Design review of the part built by this model. Coordinates are the model's own, in mm. Round coordinates to 2 decimals unless told otherwise and drop trailing zeros. Loops run counter-clockwise (first coordinate to the right, second up) from the corner with the lowest first, then second, coordinate; pieces in that order, holes last. Notation, with made-up numbers: (46.25, 60) - (96.25, 60) arc R23 cw to (96.25, 95) - close; hole circle Ø7 at (18, 7.5). An arc over 180 degrees is marked (long way). Return JSON: item names as keys, results as strings. Group by question number.
from build123d import *

# Parameters (mm, degrees)
F0_W     = 50
F0_H     = 80
F1_DEPTH = 30
F2_R     = 14.968124
F3_SIZE  = 10
F4_R     = 6
F4_R_2   = 7.5
F5_DEPTH = 80.8


with BuildPart() as f1:
    # F0 (on Top) → F1 (new body)
    with BuildSketch(Plane.XY):
        with Locations((25, -40)):
            Rectangle(F0_W, F0_H)
    extrude(amount=F1_DEPTH)

    # F2
    f2_edges = [f1.edges().sort_by_distance(p)[0] for p in [
        (50, -40, 30),
    ]]
    fillet(f2_edges, radius=F2_R)

    # F3
    f3_edges = [f1.edges().sort_by_distance(p)[0] for p in [
        (0, -40, 30),
    ]]
    chamfer(f3_edges, length=F3_SIZE)

    # F4 (on face) → F5 (cut)
    with BuildSketch(Plane.XZ.offset(80)):
        with Locations((17.158328, 19.422975)):
            Circle(F4_R)
        with Locations((32.230863, 9.653739)):
            Circle(F4_R_2)
    extrude(amount=-F5_DEPTH, mode=Mode.SUBTRACT)


solid = f1.part
Q1. Add section A-A, the plane z = 12.5. State the section outline as (x, y) points, plus the area to 3 significant figures.
Q2. Add section D-D, the plane y = -22.5. State the section outline as (x, z) points.
Q3. Draft analysis for pull direction X (two halves, no side actions). For faces 1 (the cylindrical face through (19.93, -40.56, 14.1)), 2 (the flat face through (0, -41, 10)), 3 (the flat face through (50, -41, 7)), 4 (the cylindrical face through (39.385, -40.56, 11.907)), state which applies: pulls with the +X half, pulls with the -X half, needs draft (parallel to the pull), parting line crosses it, or undercut.
Q4. Insertion check: pin 1 Ø6 at (y, z) = (-43, 23.5) entering from +X. The pin has a flat end and moves straight along its axis. Give the tip position at first contact, or say it passes through.
Q5. Add section C-C, the plane x = 27. State the section outline as (y, z) points, plus the area to 3 significant figures.
Q6. For line 1 (Z direction, x = 17, y = -30.5); line 2 (X direction, y = -41, z = 15.25); line 3 (X direction, y = -49, z = 9.5), list the stretches that pass through material, from the lowest coordinate up.
Q7. Add section B-B, the plane z = 16. State the section outline as (x, y) points.
Evaluation:
{
 "1": {"outline": "(0, -80) - (25.29, -80) - (25.29, 0) - (0, 0) - close; (39.17, -80) - (50, -80) - (50, 0) - (39.17, 0) - close", "area": "2,890 mm²"},
 "2": {"outline": "(0, 0) - (50, 0) - (50, 15.03) arc R14.97 ccw to (35.03, 30) - (10, 30) - (0, 20) - close; hole circle Ø12 at (17.16, 19.42); hole circle Ø15 at (32.23, 9.65)"},
 "3": {"face 1": "undercut", "face 2": "pulls with the -X half", "face 3": "pulls with the +X half", "face 4": "undercut"},
 "4": {"pin 1": "x = 48.97"},
 "5": {"outline": "(-80, 0) - (0, 0) - (0, 4.28) - (-80, 4.28) - close; (-80, 15.03) - (0, 15.03) - (0, 30) - (-80, 30) - close", "area": "1,540 mm²"},
 "6": {"line 1": "0 to 13.43, 25.42 to 30", "line 2": "0 to 12.85, 21.47 to 27.24, 37.22 to 50", "line 3": "0 to 24.73, 39.73 to 50"},
 "7": {"outline": "(0, -80) - (12.23, -80) - (12.23, 0) - (0, 0) - close; (22.09, -80) - (28.23, -80) - (28.23, 0) - (22.09, 0) - close; (36.23, -80) - (49.97, -80) - (49.97, 0) - (36.23, 0) - close"}
}
